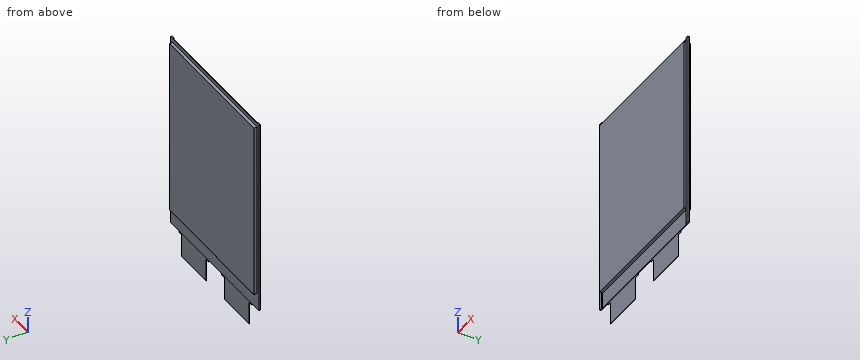
```python
from build123d import *

# Parameters (mm, degrees)
SKETCH1_W             = 153.9875
SKETCH1_H             = 203.596875
CELL_INSULATION_DEPTH = 0.3175
SKETCH1_3_W           = 153.9875
SKETCH1_3_H           = 203.596875
CELL_BODY_DEPTH       = 3.6703
CELL_BODY_DEPTH_BACK  = 3.4163
ANODE_TAB_DEPTH       = 0.1016
CATHODE_TAB_DEPTH     = 0.1397
SKETCH2_W             = 3.683
SKETCH2_H             = 227.0125
EDGE_FOLD_DEPTH       = 1.016


with BuildPart() as part:
    # Sketch1 → Cell Insulation (new body, symmetric)
    with BuildSketch(Plane(origin=(0, 0, 0), x_dir=(1, 0, 0), z_dir=(0, 1, 0))):
        Polygon((0, 227.0125), (0, 0), (161.13125, 0), (161.13125, 227.0125), (146.58975, 227.0125), (141.76375, 227.0125), (96.55175, 227.0125), (91.72575, 227.0125), (68.16725, 227.0125), (63.34125, 227.0125), (18.12925, 227.0125), (13.30325, 227.0125), align=None)
        with Locations((80.565625, 106.5609375)):
            Rectangle(SKETCH1_W, SKETCH1_H, mode=Mode.SUBTRACT)
    extrude(amount=CELL_INSULATION_DEPTH, both=True)

    # Sketch1_3 → Cell Body (add, two sides)
    with BuildSketch(Plane(origin=(0, 0, 0), x_dir=(1, 0, 0), z_dir=(0, 1, 0))) as cell_body_sk:
        with Locations((80.565625, 106.5609375)):
            Rectangle(SKETCH1_3_W, SKETCH1_3_H)
    extrude(amount=CELL_BODY_DEPTH)
    extrude(cell_body_sk.sketch, amount=-CELL_BODY_DEPTH_BACK)

    # Sketch1_4 → Anode Tab (add, symmetric)
    with BuildSketch(Plane(origin=(0, 0, 0), x_dir=(1, 0, 0), z_dir=(0, 1, 0))):
        Polygon((146.58975, 227.0125), (146.58975, 229.39375), (141.76375, 229.39375), (141.76375, 255.5875), (96.55175, 255.5875), (96.55175, 229.39375), (91.72575, 229.39375), (91.72575, 227.0125), align=None)
    extrude(amount=ANODE_TAB_DEPTH, both=True)

    # Sketch1_5 → Cathode Tab (add, symmetric)
    with BuildSketch(Plane(origin=(0, 0, 0), x_dir=(1, 0, 0), z_dir=(0, 1, 0))):
        Polygon((13.30325, 229.39375), (13.30325, 227.0125), (68.16725, 227.0125), (68.16725, 229.39375), (63.34125, 229.39375), (63.34125, 255.5875), (18.12925, 255.5875), (18.12925, 229.39375), align=None)
    extrude(amount=CATHODE_TAB_DEPTH, both=True)

    # Sketch2 → Edge Fold (add)
    with BuildSketch(Plane.XZ.offset(0.3175)):
        with Locations((1.8415, -113.50625)):
            Rectangle(SKETCH2_W, SKETCH2_H)
    edge_fold = extrude(amount=EDGE_FOLD_DEPTH)

    # Edge Folds Mirror: Edge Fold across plane
    add(edge_fold.mirror(Plane.ZY.offset(-80.565625)))


solid = part.part
```
Could you check a few things on this model? Use its own coordinates, in mm. Give positions to 0.01 mm unless a question says otherwise; leave off trailing zeros. Loops run counter-clockwise (first coordinate to the right, second up) from the corner with the lowest first, then second, coordinate; pieces in that order, holes last. Notation, with made-up numbers: (5.5, -21.75) - (40.5, -21.75) arc R25 ccw to (40.5, 12.25) - close; hole circle Ø2 at (-7.5, -18.5). An arc over 180 degrees is marked (long way). Answer in a Markdown table with one row per item. Add a question column.
Q1. If we section it at D-D (z = -22.5): List the corners of the cut face in (x, y) for me, plus the area to 3 significant figures.
Q2. Please list where these lines run through material, in increasing order: L1, parallel to X at y = 3, z = -17.5; L2, parallel to Z at x = 39, y = -0.5; L3, parallel to Z at x = 112.5, y = -0.25. Write a range as from..to.
Q3. For pin 1 (1 mm diameter, centred on y = 2, z = -77, fed in from -X); pin 2 (5 mm diameter, centred on x = 124, z = -228, fed in from +Y); pin 3 (4 mm diameter, centred on x = 61, y = 2.5, fed in from -Z); pin 4 (1 mm diameter, centred on y = -1, z = -229, fed in from -X), each with a flat end and sliding along its axis, tell me the tip position at first contact or that it passes through.
Q4. If we section it at B-B (x = 135.5): List the corners of the cut face in (y, z) for me.
Q5. If we section it at A-A (z = -232): List the corners of the cut face in (x, y) for me.
Q6. If we section it at C-C (y = 2.5): List the corners of the cut face in (x, z) for me.
The answers:
| question | item | result |
|---|---|---|
| 1 | outline | (0, -1.33) - (3.57, -1.33) - (3.57, -3.42) - (157.56, -3.42) - (157.56, -1.33) - (161.13, -1.33) - (161.13, 0.32) - (157.56, 0.32) - (157.56, 3.67) - (3.57, 3.67) - (3.57, 0.32) - (0, 0.32) - close |
| 1 | area | 1,100 mm^2 |
| 2 | L1 | x = 3.57..157.56 |
| 2 | L2 | z = -208.36..-4.76 |
| 2 | L3 | z = -227.01..0 |
| 3 | pin 1 | stops at x = 3.57 |
| 3 | pin 2 | stops at y = 0.32 |
| 3 | pin 3 | stops at z = -208.36 |
| 3 | pin 4 | passes through |
| 4 | outline | (-3.42, -208.36) - (-0.32, -208.36) - (-0.32, -227.01) - (-0.1, -227.01) - (-0.1, -255.59) - (0.1, -255.59) - (0.1, -227.01) - (0.32, -227.01) - (0.32, -208.36) - (3.67, -208.36) - (3.67, -4.76) - (0.32, -4.76) - (0.32, 0) - (-0.32, 0) - (-0.32, -4.76) - (-3.42, -4.76) - close |
| 5 | outline | (18.13, -0.14) - (63.34, -0.14) - (63.34, 0.14) - (18.13, 0.14) - close; (96.55, -0.1) - (141.76, -0.1) - (141.76, 0.1) - (96.55, 0.1) - close |
| 6 | outline | (3.57, -208.36) - (157.56, -208.36) - (157.56, -4.76) - (3.57, -4.76) - close |
